CAD build for the part. Positions are in the model's coordinates, mm. A direction names the side the tool comes from. Give positions to 0.01 mm unless a question says otherwise; leave off trailing zeros. Loops run counter-clockwise (first coordinate to the right, second up) from the corner with the lowest first, then second, coordinate; pieces in that order, holes last. Notation, with made-up numbers: (73, 75) -> (96, 75) arc R29 ccw to (96, 108) -> close; hole circle Ø2 at (55.5, 29.25). An arc over 180 degrees is marked (long way). Use one line per item in the form item = value.
```python
from build123d import *

# Parameters (mm, degrees)
BOSS_EXTRUDE5_DEPTH = 40
FILLET4_RADIUS      = 20
FILLET4_LENGTH      = 15
SKETCH8_R           = 14
CUT_EXTRUDE1_DEPTH  = 40
SKETCH9_R           = 4
CUT_EXTRUDE2_DEPTH  = 40


with BuildPart() as part:
    # Sketch1 → Boss-Extrude5 (new body)
    with BuildSketch(Plane.XY):
        Polygon((-36, 44), (-36, -13), (0, -13), (0, 0), (-21, 0), (-21, 44), align=None)
    extrude(amount=BOSS_EXTRUDE5_DEPTH)

    # Fillet4: full round fillet: the end face becomes a half cylinder, R = half its width
    fillet4_face = Plane((-28.5, 44, 20), x_dir=(1, 0, 0), z_dir=(0, 1, 0))  # on the end face: x along it, z out of the body
    fillet4_slab = fillet4_face.offset(-FILLET4_RADIUS / 2) * Box(FILLET4_LENGTH, 2 * FILLET4_RADIUS, FILLET4_RADIUS, mode=Mode.PRIVATE)  # the body's end, R deep
    fillet4_round = Plane((-28.5, 24, 20), x_dir=(0, 1, 0), z_dir=(1, 0, 0)) * Cylinder(FILLET4_RADIUS, FILLET4_LENGTH, mode=Mode.PRIVATE)  # its axis R under the face
    add(fillet4_slab - fillet4_round, mode=Mode.SUBTRACT)

    # Sketch8 → Cut-Extrude1 (cut)
    with BuildSketch(Plane(origin=(-21, 0, 0), x_dir=(0, 0, -1), z_dir=(1, 0, 0))):
        with Locations((-20, 22)):
            Circle(SKETCH8_R)
    extrude(amount=-CUT_EXTRUDE1_DEPTH, mode=Mode.SUBTRACT)

    # Sketch9 → Cut-Extrude2 (cut)
    with BuildSketch(Plane(origin=(0, 0, 0), x_dir=(1, 0, 0), z_dir=(0, 1, 0))):
        with Locations(Location((-11, -10, 0), (0, 0, 180))):
            Circle(SKETCH9_R)
        with Locations(Location((-11, -30, 0), (0, 0, 180))):
            Circle(SKETCH9_R)
    extrude(amount=-CUT_EXTRUDE2_DEPTH, mode=Mode.SUBTRACT)


solid = part.part
```
1. Cut at C-C, the plane z = 19. Write the cut outline in (x, y).
Result sheet:
outline = (-36, -13) -> (0, -13) -> (0, 0) -> (-21, 0) -> (-21, 8.04) -> (-36, 8.04) -> close; (-36, 35.96) -> (-21, 35.96) -> (-21, 43.97) -> (-36, 43.97) -> close
2. Cut at D-D, the plane x = -22. Write the cut outline in (y, z).
Result sheet:
outline = (-13, 0) -> (24, 0) arc R20 ccw to (24, 40) -> (-13, 40) -> close; hole circle Ø28 at (22, 20)
3. Cut at A-A, the plane y = 22. Write the cut outline in (x, z).
Result sheet:
outline = (-36, 0) -> (-21, 0) -> (-21, 6) -> (-36, 6) -> close; (-36, 34) -> (-21, 34) -> (-21, 40) -> (-36, 40) -> close
4. Mould opens along X. For faces 1 (the flat face through (-18, -13, 20)), 2 (the cylindrical face through (-10.479, -6.409, 33.966)), 3 (the cylindrical face through (-8.05, -6.41, 12.7)), 4 (the flat face through (-21, 7, 20)) say: pulls with the +X half, pulls with the -X half, needs draft (parallel to the pull), parting line crosses it, or undercut.
Result sheet:
face_1 = needs draft
face_2 = undercut
face_3 = undercut
face_4 = pulls with the +X half
5. Cut at B-B, the plane x = -13. Write the cut outline in (y, z).
Result sheet:
outline = (-13, 0) -> (0, 0) -> (0, 6.54) -> (-13, 6.54) -> close; (-13, 13.46) -> (0, 13.46) -> (0, 26.54) -> (-13, 26.54) -> close; (-13, 33.46) -> (0, 33.46) -> (0, 40) -> (-13, 40) -> close
6. Drop flat-ended pins along their axis: P1, Ø6, axis at x = -6, y = -2, coming from the -Z side; P2, Ø6.5, axis at x = -11.5, z = 14.5, coming from the +Y side; P3, Ø6, axis at x = -23, y = 31, coming from the +Z side; P4, Ø12, axis at y = 28, z = 29, coming from the +X side. Give the stop position or say it passes through.
Result sheet:
P1 = 0
P2 = 0
P3 = 39.6
P4 = -21
7. Tool access for faces 5 (the flat face through (-10, 0, 20)), 6 (the flat face through (-22, 2, 40)): list every direction of +Z, -Z, +X, -X, +Y, -Y with a clear straight run to the whole face (end or side of a thin tool).
Result sheet:
face_5 = +Z, -Z, +X, +Y
face_6 = +Z, +X, -X, +Y, -Y
8. Drill centre lines: line 1 (Z direction, x = -11, y = -4.5); line 2 (X direction, y = 36.5, z = 34); line 3 (Y direction, x = -33, z = 22). Where is each one in solid material? Low to high.
Result sheet:
line_1 = 0 to 6, 14 to 26, 34 to 40
line_2 = -36 to -21
line_3 = -13 to 8.14, 35.86 to 43.9
